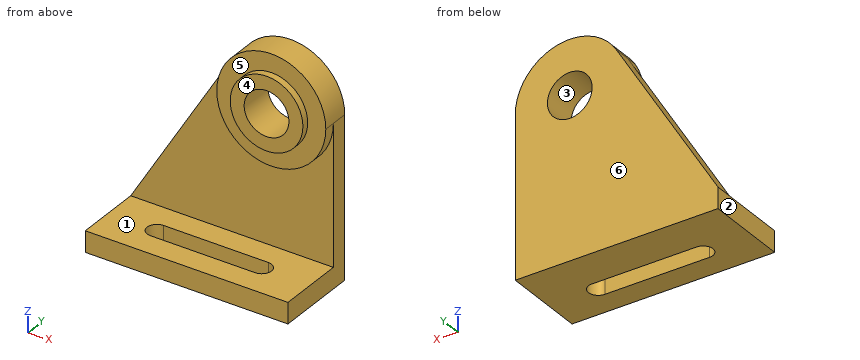
from build123d import *

# Parameters (mm, degrees)
F0_R     = 26
F0_R_2   = 16
F1_DEPTH = 25
F2_DEPTH = 20
F3_DEPTH = 12
F0_W     = 145
F0_H     = 15
F4_DEPTH = 60
F6_DEPTH = 25


with BuildPart() as f1:
    # F0 (on Front) → F1 (new body)
    with BuildSketch(Plane.XZ):
        with Locations((23.226776, 54.015426)):
            Circle(F0_R)
        with Locations((23.226776, 54.015426)):
            Circle(F0_R_2, mode=Mode.SUBTRACT)
    extrude(amount=F1_DEPTH)

    # F0 (on Front) → F2 (join)
    with BuildSketch(Plane.XZ):
        with BuildLine():
            ThreePointArc((62.226776, 54.015426), (33.696714, 91.583769), (-10.151705, 74.186617))
            ThreePointArc((-10.151705, 74.186617), (12.756838, 16.447083), (62.226776, 54.015426))
        make_face()
        with Locations((23.226776, 54.015426)):
            Circle(F0_R, mode=Mode.SUBTRACT)
    extrude(amount=F2_DEPTH)

    # F0 (on Front) → F3 (join)
    with BuildSketch(Plane.XZ):
        with BuildLine():
            Line((-10.151705, 74.186617), (-82.773224, -45.984574))
            Line((-82.773224, -45.984574), (62.226776, -45.984574))
            Line((62.226776, -45.984574), (62.226776, 54.015426))
            ThreePointArc((62.226776, 54.015426), (12.756838, 16.447083), (-10.151705, 74.186617))
        make_face()
    extrude(amount=F3_DEPTH)

    # F0 (on Front) → F4 (join)
    with BuildSketch(Plane.XZ):
        with Locations((-10.273224, -53.484574)):
            Rectangle(F0_W, F0_H)
    extrude(amount=F4_DEPTH)

    # F5 (on face) → F6 (cut)
    with BuildSketch(Plane.XY.offset(-45.984574)):
        with BuildLine():
            Line((27.226776, -29), (-47.773224, -29))
            ThreePointArc((-47.773224, -29), (-54.773224, -36), (-47.773224, -43))
            Line((-47.773224, -43), (27.226776, -43))
            ThreePointArc((27.226776, -43), (34.226776, -36), (27.226776, -29))
        make_face()
    extrude(amount=-F6_DEPTH, mode=Mode.SUBTRACT)


solid = f1.part
Source: CAD feature listing. Evaluate the final solid. Frame: model axes, mm. Face numbers are marked on the shaded views. A direction names the side the tool comes from. Give positions to 0.01 mm unless a question says otherwise; leave off trailing zeros. Write each loop counter-clockwise with the first axis right and the second up, starting at its lowest first coordinate (ties: lowest second). Pieces come first, ordered by that corner, then holes. Notation, with made-up numbers: M 81.25,85 L 128.25,85 A18 cw 128.25,94 Z; hole C 50,73 d6. An arc over 180 degrees is marked long. Return JSON: item names as keys, results as strings. Group by question number.
1) First-contact query: pin 1 Ø12 at (x, z) = (43, -26) entering from -Y; pin 2 Ø4.5 at (x, z) = (-20.5, -51.5) entering from +Y; pin 3 Ø14.5 at (x, y) = (12.5, -30) entering from +Z; pin 4 Ø15.5 at (x, z) = (14, 48) entering from -Y. Flat tips, straight axial feed; report the tip coordinate or a pass-through.
2) Cut plane C-C, the plane x = -12.5. Output: boundary loops of the cut face in (y, z).
3) Cut plane A-A, the plane y = -9.5. Output: boundary loops of the cut face in (x, z), then the cut area to 3 significant figures.
4) Cut plane D-D, the plane z = 77. Output: boundary loops of the cut face in (x, y).
5) Cut plane B-B, the plane y = -36. Output: boundary loops of the cut face in (x, z).
6) Set-up query: the marked faces 4, 5 and 6. Return all of +Z, -Z, +X, -X, +Y, -Y with unobstructed straight access to the full face (end or side cutting, diameter ignored); none if empty.
7) Draft query along X for the marked faces 1, 2 and 3. Return one class per face: released by +X, released by -X, zero draft, split by the parting line, or undercut.
8) Ray query, L1, parallel to Y at x = -44, z = -50; L2, parallel to Y at x = 12.5, z = 33.5; L3, parallel to Z at x = -59.5, y = -25. Return the intervals inside material, ascending.
Data:
{
 "1": {"pin 1": "stops at y = -12", "pin 2": "stops at y = 0", "pin 3": "stops at z = 79.43", "pin 4": "stops at y = -25"},
 "2": {"outline": "M -60,-60.98 L -43,-60.98 L -43,-45.98 L -60,-45.98 Z; M -29,-60.98 L 0,-60.98 L 0,70.3 L -12,70.3 L -12,69.66 L -20,69.66 L -20,38.38 L -12,38.38 L -12,-45.98 L -29,-45.98 Z"},
 "3": {"outline": "M -82.77,-60.98 L 62.23,-60.98 L 62.23,54.02 A39 ccw -10.15,74.19 L -82.77,-45.98 Z; hole C 23.23,54.02 d32", "area": "15,300 mm²"},
 "4": {"outline": "M -8.28,-20 L 11.07,-20 L 11.07,-25 L 35.38,-25 L 35.38,-20 L 54.73,-20 L 54.73,0 L -8.28,0 Z"},
 "5": {"outline": "M -82.77,-60.98 L -54.77,-60.98 L -54.77,-45.98 L -82.77,-45.98 Z; M 34.23,-60.98 L 62.23,-60.98 L 62.23,-45.98 L 34.23,-45.98 Z"},
 "6": {"face 4": "+Z, +X, -X, -Y", "face 5": "-Y", "face 6": "+Z, -Z, +X, -X, +Y"},
 "7": {"face 1": "zero draft", "face 2": "released by -X", "face 3": "undercut"},
 "8": {"L1": "y = -60 to -43, -29 to 0", "L2": "y = -25 to 0", "L3": "z = -60.98 to -45.98"}
}
